The listing builds one solid part. Answer for the finished solid, in the listing's coordinates (mm). A direction names the side the tool comes from. Coordinates: 2 decimals unless noted, no trailing zeros. Order: outer loops, then holes, each group sorted by start corner. A loop starts at its lowest first (then second) coordinate and runs counter-clockwise, first axis right, second up. Notation, with made-up numbers: (-21, -11.75) -> (30, -11.75) arc R35 ccw to (30, 27.25) -> close; hole circle Ø7 at (-31.5, -16.75). An arc over 180 degrees is marked (long way). Return JSON: item names as keys, results as strings.
```python
from build123d import *

# Parameters (mm, degrees)
SKETCH1_R           = 7.925000025
BOSS_EXTRUDE1_DEPTH = 58.000000078
SKETCH2_R           = 7.899999948
BOSS_EXTRUDE2_DEPTH = 4
SKETCH3_R           = 7.925000025
BOSS_EXTRUDE3_DEPTH = 37.7
SKETCH4_W           = 3.302
SKETCH4_H           = 27.5
CUT_EXTRUDE1_DEPTH  = 2.032
CIRPATTERN1_COUNT   = 6
SKETCH10_W          = 1
SKETCH10_H          = 17
CUT_EXTRUDE2_DEPTH  = 0.75
CIRPATTERN2_COUNT   = 24


with BuildPart() as part:
    # Sketch1 → Boss-Extrude1 (new body)
    with BuildSketch(Plane.XY):
        Circle(SKETCH1_R)
    extrude(amount=BOSS_EXTRUDE1_DEPTH)

    # Sketch2 → Boss-Extrude2 (add)
    with BuildSketch(Plane.XY.offset(58.000000078)):
        Circle(SKETCH2_R)
    extrude(amount=BOSS_EXTRUDE2_DEPTH)

    # Sketch3 → Boss-Extrude3 (add)
    with BuildSketch(Plane.XY.offset(62.000000078)):
        Circle(SKETCH3_R)
    extrude(amount=BOSS_EXTRUDE3_DEPTH)

    # Sketch4 → Cut-Extrude1 (cut)
    with BuildSketch(Plane(origin=(0, 7.925000025, 0), x_dir=(1, 0, 0), z_dir=(0, 1, 0))):
        with Locations((0, -85.950000078)):
            Rectangle(SKETCH4_W, SKETCH4_H)
    cut_extrude1 = extrude(amount=-CUT_EXTRUDE1_DEPTH, mode=Mode.SUBTRACT)

    # CirPattern1: Cut-Extrude1 ×6 about axis
    cirpattern1_axis = Axis((0, 0, 0), (0, 0, 1))
    for i in range(1, CIRPATTERN1_COUNT):
        add(cut_extrude1.rotate(cirpattern1_axis, i * 360 / CIRPATTERN1_COUNT), mode=Mode.SUBTRACT)

    # Sketch10 → Cut-Extrude2 (cut)
    with BuildSketch(Plane(origin=(0, 7.925000025, 0), x_dir=(1, 0, 0), z_dir=(0, 1, 0))):
        with Locations((0, -8.5)):
            Rectangle(SKETCH10_W, SKETCH10_H)
    cut_extrude2 = extrude(amount=-CUT_EXTRUDE2_DEPTH, mode=Mode.SUBTRACT)

    # CirPattern2: Cut-Extrude2 ×24 about axis
    cirpattern2_axis = Axis((0, 0, 0), (0, 0, 1))
    for i in range(1, CIRPATTERN2_COUNT):
        add(cut_extrude2.rotate(cirpattern2_axis, i * 360 / CIRPATTERN2_COUNT), mode=Mode.SUBTRACT)


solid = part.part
```
Item 1: Which of the six approach directions +Z, -Z, +X, -X, +Y, -Y give full straight-line access (tool end or side, diameter ignored) to faces 1 (the flat face through (6, -3, 72.2)), 2 (the flat face through (-5.094, 4.847, 86.143)), 3 (the flat face through (-6.745, 1.988, 86.143))?
Answer list:
{"face 1": "+Z", "face 2": "+Z, -X", "face 3": "+Z, +Y"}
Item 2: The part is cut by section A-A on z = 90.5. Determine the outline of the cut face in (x, y) (3 decimals), plus the area to 3 significant figures.
Answer list:
{"outline": "(-7.538, -2.446) -> (-5.929, -1.517) -> (-4.278, -4.376) -> (-5.887, -5.305) arc R7.925 ccw to (-1.651, -7.751) -> (-1.651, -5.893) -> (1.651, -5.893) -> (1.651, -7.751) arc R7.925 ccw to (5.887, -5.305) -> (4.278, -4.376) -> (5.929, -1.517) -> (7.538, -2.446) arc R7.925 ccw to (7.538, 2.446) -> (5.929, 1.517) -> (4.278, 4.376) -> (5.887, 5.305) arc R7.925 ccw to (1.651, 7.751) -> (1.651, 5.893) -> (-1.651, 5.893) -> (-1.651, 7.751) arc R7.925 ccw to (-5.887, 5.305) -> (-4.278, 4.376) -> (-5.929, 1.517) -> (-7.538, 2.446) arc R7.925 ccw to start", "area": "158 mm2"}
Item 3: Flat-ended cylindrical pins translate along their axes: pin 1 (5 mm diameter, centred on y = -3, z = 35, fed in from -X); pin 2 (1 mm diameter, centred on x = -3.5, z = 40.5, fed in from +Y); pin 3 (1 mm diameter, centred on x = -6, y = -4, fed in from +Z). Find the tip coordinate at first contact, or state that the pin passes through.
Answer list:
{"pin 1": "x = -7.91", "pin 2": "y = 7.34", "pin 3": "z = 72.2"}
Item 4: Determine the mould class of faces 4 (the cylindrical face through (-7.917, 0.348, 80.586)), 5 (the flat face through (0, -5.893, 86)), 6 (the flat face through (-5.094, -4.847, 86.143)) for opening direction Y: pulls with the +Y half, pulls with the -Y half, needs draft (parallel to the pull), parting line crosses it, or undercut.
Answer list:
{"face 4": "parting line crosses it", "face 5": "pulls with the -Y half", "face 6": "undercut"}
Item 5: The part is cut by section B-B on z = 33. Determine the outline of the cut face in (x, y) (3 decimals).
Answer list:
{"outline": "circle Ø15.85 at (0, 0)"}
Item 6: Find the intervals of material crossed by probe 1 along Y at (x, z) = (5.75, 79); probe 2 along Y at (x, z) = (-5, 6.5); probe 3 along Y at (x, z) = (0.25, 29.5), in increasing order.
Answer list:
{"probe 1": "-5.45 to -5.23, -1.83 to 1.83, 5.23 to 5.45", "probe 2": "-6.15 to -5.71, -5.15 to 5.15, 5.71 to 6.15", "probe 3": "-7.92 to 7.92"}
